```python
from build123d import *

# Parameters (mm, degrees)
BOSS_EXTRUDE1_DEPTH = 6
BOSS_EXTRUDE2_DEPTH = 5
SKETCH2_W           = 3
SKETCH2_H           = 13.7
CUT_EXTRUDE1_DEPTH  = 7


with BuildPart() as part:
    # Sketch1 → Boss-Extrude1 (new body)
    with BuildSketch(Plane(origin=(0, 0, 0), x_dir=(1, 0, 0), z_dir=(0, 1, 0))):
        with BuildLine():
            ThreePointArc((-54.157142857, -25.121581908), (59.7, 0), (-54.157142857, 25.121581908))
            ThreePointArc((-54.157142857, 25.121581908), (-99.7, 0), (-54.157142857, -25.121581908))
        make_face()
    extrude(amount=BOSS_EXTRUDE1_DEPTH)

    # Sketch1<3> → Boss-Extrude2 (add)
    with BuildSketch(Plane(origin=(0, 0, 0), x_dir=(1, 0, 0), z_dir=(0, 1, 0))):
        with BuildLine():
            ThreePointArc((-56.728571429, -33.141502435), (65.7, 0), (-56.728571429, 33.141502435))
            ThreePointArc((-56.728571429, 33.141502435), (-105.7, 0), (-56.728571429, -33.141502435))
        make_face()
        with BuildLine():
            ThreePointArc((-54.157142857, -25.121581908), (59.7, 0), (-54.157142857, 25.121581908))
            ThreePointArc((-54.157142857, 25.121581908), (-99.7, 0), (-54.157142857, -25.121581908))
        make_face(mode=Mode.SUBTRACT)
    extrude(amount=BOSS_EXTRUDE2_DEPTH)

    # Sketch2 → Cut-Extrude1 (cut, through all)
    with BuildSketch(Plane(origin=(0, 6, 0), x_dir=(1, 0, 0), z_dir=(0, 1, 0))):
        with Locations((39.508087625, -0.596031436)):
            Rectangle(SKETCH2_W, SKETCH2_H)
    extrude(amount=-CUT_EXTRUDE1_DEPTH, mode=Mode.SUBTRACT)


solid = part.part
```
Work out the finished part from the listing and answer in its coordinate system (mm). A direction names the side the tool comes from. Give positions to 0.01 mm unless a question says otherwise; leave off trailing zeros. Order: outer loops, then holes, each group sorted by start corner. A loop starts at its lowest first (then second) coordinate and runs counter-clockwise, first axis right, second up.
1. Section A-A, the plane x = -70 is taken. Determine the outline of the cut face in (y, z).
Result sheet:
outline: (0, -35.7) - (5, -35.7) - (5, -29.7) - (6, -29.7) - (6, 29.7) - (5, 29.7) - (5, 35.7) - (0, 35.7) - close
2. Each of these flat-tipped pins is pushed along its axis until it touches: P1, Ø2.5, axis at x = 39.5, y = 4.5, coming from the +Z side; P2, Ø1, axis at y = 4, z = -19, coming from the -X side; P3, Ø1, axis at y = 1.5, z = 45.5, coming from the +X side. Where does it stop, or does it pass through?
Result sheet:
P1: stops at z = 53.42
P2: stops at x = -100.53
P3: stops at x = 47.87
3. Straight lines are drawn through the part: L1, parallel to X at y = 3.4, z = 1.5; L2, parallel to Y at x = 58.5, z = 22; L3, parallel to Z at x = 0, y = 1.5. For each, find the intervals that lie inside material, in ascending order.
Result sheet:
L1: x = -105.67 to 38.01, 41.01 to 65.68
L2: y = 0 to 5
L3: z = -65.7 to 65.7
4. The mould has two halves that part along Z. Classify faces 4 (the cylindrical face through (59.657, 5.493, 2.262)), 5 (the flat face through (38.008, 3, 1)), 6 (the flat face through (-21, 6, -1)): released by +Z, released by -Z, zero draft, split by the parting line, or undercut.
Result sheet:
face 4: split by the parting line
face 5: undercut
face 6: zero draft
5. For faces 1 (the flat face through (-52, 5, -30)), 2 (the flat face through (-21, 0, -1)), 3 (the flat face through (41.008, 3, 1)), determine the directions among +Z, -Z, +X, -X, +Y, -Y from which every point of the face is accessible in a straight line to the end or side of a thin tool.
Result sheet:
face 1: +Y
face 2: +Z, -Z, +X, -X, -Y
face 3: +Y, -Y
6. Section B-B, the plane z = -45 is taken. Determine the outline of the cut face in (x, y), and give its area (3 significant figures).
Result sheet:
outline: (-47.87, 0) - (47.87, 0) - (47.87, 5) - (39.23, 5) - (39.23, 6) - (-39.23, 6) - (-39.23, 5) - (-47.87, 5) - close
area: 557 mm2
